Check sheet for the modelled part. Datum: model origin and axes. Units: mm. A direction names the side the tool comes from. Round coordinates to 2 decimals unless told otherwise and drop trailing zeros. Write each loop counter-clockwise with the first axis right and the second up, starting at its lowest first coordinate (ties: lowest second). Pieces come first, ordered by that corner, then holes. Notation, with made-up numbers: (77.25, 70.25) -> (123.25, 70.25) arc R12 cw to (123.25, 88.25) -> close; hole circle Ø3 at (80, 35). An arc over 180 degrees is marked (long way). Put each result on its own line as item: value. Start each with the question number.
from build123d import *

# Parameters (mm, degrees)
BOSS_EXTRUDE3_DEPTH = 150
SKETCH6_R           = 12.5
CUT_EXTRUDE3_DEPTH  = 50
SKETCH7_R           = 25
CUT_EXTRUDE4_DEPTH  = 20
SKETCH8_R           = 12.5
CUT_EXTRUDE7_DEPTH  = 50
SKETCH11_R          = 25
CUT_EXTRUDE8_DEPTH  = 20
SKETCH12_R          = 25
CUT_EXTRUDE9_DEPTH  = 150
SKETCH14_W          = 40
SKETCH14_H          = 200
CUT_EXTRUDE10_DEPTH = 65
SKETCH15_W          = 70
SKETCH15_H          = 200
CUT_EXTRUDE11_DEPTH = 100
CUT_EXTRUDE12_DEPTH = 110


with BuildPart() as part:
    # Sketch2 → Boss-Extrude3 (new body)
    with BuildSketch(Plane(origin=(0, 0, 0), x_dir=(1, 0, 0), z_dir=(0, 1, 0))):
        with BuildLine():
            Line((0, 0), (0, 200))
            Line((0, 200), (225, 200))
            Line((225, 200), (280, 142.246569699))
            Line((280, 142.246569699), (334.500730705, 142.246569699))
            ThreePointArc((334.500730705, 142.246569699), (395, 100), (334.500730705, 57.753430301))
            Line((334.500730705, 57.753430301), (280, 57.753430301))
            Line((280, 57.753430301), (225, 0))
            Line((225, 0), (0, 0))
        make_face()
    extrude(amount=BOSS_EXTRUDE3_DEPTH)

    # Sketch6 → Cut-Extrude3 (cut)
    with BuildSketch(Plane.XZ):
        with Locations(Location((75.424439909, -45, 0), (0, 0, 270))):
            Circle(SKETCH6_R)
    extrude(amount=-CUT_EXTRUDE3_DEPTH, mode=Mode.SUBTRACT)

    # Sketch7 → Cut-Extrude4 (cut)
    with BuildSketch(Plane.XZ):
        with Locations(Location((75.424439909, -45, 0), (0, 0, 270))):
            Circle(SKETCH7_R)
    extrude(amount=-CUT_EXTRUDE4_DEPTH, mode=Mode.SUBTRACT)

    # Sketch8 → Cut-Extrude7 (cut)
    with BuildSketch(Plane.XZ):
        with Locations(Location((75, -155, 0), (0, 0, 270))):
            Circle(SKETCH8_R)
    extrude(amount=-CUT_EXTRUDE7_DEPTH, mode=Mode.SUBTRACT)

    # Sketch11 → Cut-Extrude8 (cut)
    with BuildSketch(Plane(origin=(0, 0, 0), x_dir=(-1, 0, 0), z_dir=(0, -1, 0))):
        with Locations(Location((-75, 155, 0), (0, 0, 90))):
            Circle(SKETCH11_R)
    extrude(amount=-CUT_EXTRUDE8_DEPTH, mode=Mode.SUBTRACT)

    # Sketch12 → Cut-Extrude9 (cut)
    with BuildSketch(Plane(origin=(0, 0, 0), x_dir=(-1, 0, 0), z_dir=(0, -1, 0))):
        with Locations(Location((-350, 99.787780046, 0), (0, 0, 90))):
            Circle(SKETCH12_R)
    extrude(amount=-CUT_EXTRUDE9_DEPTH, mode=Mode.SUBTRACT)

    # Sketch14 → Cut-Extrude10 (cut)
    with BuildSketch(Plane(origin=(0, 150, 0), x_dir=(1, 0, 0), z_dir=(0, 1, 0))):
        with Locations((20, 100)):
            Rectangle(SKETCH14_W, SKETCH14_H)
    extrude(amount=-CUT_EXTRUDE10_DEPTH, mode=Mode.SUBTRACT)

    # Sketch15 → Cut-Extrude11 (cut)
    with BuildSketch(Plane(origin=(0, 150, 0), x_dir=(1, 0, 0), z_dir=(0, 1, 0))):
        with Locations((75, 100)):
            Rectangle(SKETCH15_W, SKETCH15_H)
    extrude(amount=-CUT_EXTRUDE11_DEPTH, mode=Mode.SUBTRACT)

    # Sketch16 → Cut-Extrude12 (cut)
    with BuildSketch(Plane.XZ):
        with BuildLine():
            Line((150, -200), (150, 0))
            Line((150, 0), (225, 0))
            Line((225, 0), (280, -57.753430301))
            Line((280, -57.753430301), (334.500730705, -57.753430301))
            ThreePointArc((334.500730705, -57.753430301), (395, -100), (334.500730705, -142.246569699))
            Line((334.500730705, -142.246569699), (280, -142.246569699))
            Line((280, -142.246569699), (225, -200))
            Line((225, -200), (150, -200))
        make_face()
    extrude(amount=-CUT_EXTRUDE12_DEPTH, mode=Mode.SUBTRACT)


solid = part.part
1. Section check D-D, the plane x = 81. Enter the section's corners in (y, z), then the cut area to 3 significant figures.
2. Material ranges on L1, parallel to X at y = 7.75, z = -155; L2, parallel to X at y = 31, z = -155; L3, parallel to Y at x = 225.5, z = -156, recorded low to high. Write a range as [from, to].
3. Section check C-C, the plane z = -100. Enter the section's corners in (x, y).
4. Gauge pin test, flat ends, axial feed: P1, Ø10.5, axis at y = 64, z = -118.5, coming from the +X side; P2, Ø1, axis at x = 44, z = -144.5, coming from the +Y side; P3, Ø1, axis at x = 221.5, z = -37, coming from the -Y side; P4, Ø22.5, axis at x = 75, z = -155, coming from the +Y side. Record the tip position at first contact, or that the pin passes through.
5. Draft check along Z on faces 4 (the flat face through (110, 101, -99)), 5 (the flat face through (81.3, 20, -33.5)), 6 (the flat face through (252.885, 129.72, -29.281)). Enter one of: released by +Z, released by -Z, zero draft, split by the parting line, or undercut.
6. Section check A-A, the plane x = 350. Enter the section's corners in (y, z), then the cut area to 3 significant figures.
7. Access from +Z, -Z, +X, -X, +Y, -Y to the whole of each face (thin tool, end or side, straight path). Record for faces 1 (the flat face through (307, 130, -142.247)), 2 (the flat face through (247, 110, -99)), 3 (the cylindrical face through (92.321, 9.86, -26.574)).
8. Section check B-B, the plane y = 62.5. Enter the section's corners in (x, z).
Reply:
1. outline: (0, -200) -> (50, -200) -> (50, -165.97) -> (20, -165.97) -> (20, -179.27) -> (0, -179.27) -> close; (0, -130.73) -> (20, -130.73) -> (20, -144.03) -> (50, -144.03) -> (50, -56.19) -> (20, -56.19) -> (20, -69.37) -> (0, -69.37) -> close; (0, -20.63) -> (20, -20.63) -> (20, -33.81) -> (50, -33.81) -> (50, 0) -> (0, 0) -> close
1. area: 6,730 mm2
2. L1: x = [0, 50], [100, 150]
2. L2: x = [0, 62.5], [87.5, 150]
2. L3: y = [110, 150]
3. outline: (0, 0) -> (150, 0) -> (150, 110) -> (325, 110) -> (325, 150) -> (110, 150) -> (110, 50) -> (40, 50) -> (40, 85) -> (0, 85) -> close; (375, 110) -> (395, 110) -> (395, 150) -> (375, 150) -> close
4. P1: stops at x = 150
4. P2: stops at y = 50
4. P3: stops at y = 110
4. P4: passes through
5. face 4: zero draft
5. face 5: undercut
5. face 6: released by +Z
6. outline: (110, -145) -> (150, -145) -> (150, -124.79) -> (110, -124.79) -> close; (110, -74.79) -> (150, -74.79) -> (150, -55) -> (110, -55) -> close
6. area: 1,600 mm2
7. face 1: -Z, +Y, -Y
7. face 2: +Z, -Z, +X, -Y
7. face 3: -Y
8. outline: (0, -200) -> (40, -200) -> (40, 0) -> (0, 0) -> close; (110, -200) -> (150, -200) -> (150, 0) -> (110, 0) -> close
